```python
from build123d import *

# Parameters (mm, degrees)
F0_R      = 15.5
F1_DEPTH  = 57.2
F3_DEPTH  = 58.1
F4_R      = 9.45
F5_DEPTH  = 3.5
F5_FACE_R = 9.45
F6_DEPTH  = 34
F7_R      = 4
F8_DEPTH  = 16
F9_R      = 4
F9_R_2    = 2
F10_DEPTH = 2
F11_DEPTH = 29
F12_R     = 6
F13_DEPTH = 2


with BuildPart() as f1:
    # F0 (on Top) → F1 (new body)
    with BuildSketch(Plane.XY):
        Circle(F0_R)
    extrude(amount=F1_DEPTH)

    # F2 (on face) → F3 (join)
    with BuildSketch(Plane.XY.offset(57.2)):
        with BuildLine():
            Line((-12.208501, 9.55), (-20.06, 9.55))
            Line((-20.06, 9.55), (-20.06, -17.45))
            Line((-20.06, -17.45), (20.06, -17.45))
            Line((20.06, -17.45), (20.06, 9.55))
            Line((20.06, 9.55), (12.208501, 9.55))
            ThreePointArc((12.208501, 9.55), (14.65404, 5.050655), (15.5, 0))
            ThreePointArc((15.5, 0), (-5.050655, -14.65404), (-12.208501, 9.55))
        make_face()
        with BuildLine():
            Line((12.208501, 9.55), (-12.208501, 9.55))
            ThreePointArc((-12.208501, 9.55), (-5.050655, -14.65404), (15.5, 0))
            ThreePointArc((15.5, 0), (14.65404, 5.050655), (12.208501, 9.55))
        make_face()
    extrude(amount=F3_DEPTH)

    # F4 (on face) → F5 (join)
    with BuildSketch(Plane.XZ.offset(17.45)):
        with Locations((0, 95.1)):
            Circle(F4_R)
    extrude(amount=F5_DEPTH)

    # F5_face (on face) → F6 (join)
    with BuildSketch(Plane(origin=(0, -20.95, 95.1), x_dir=(1, 0, 0), z_dir=(0, -1, 0))):
        Circle(F5_FACE_R)
    extrude(amount=-F6_DEPTH)

    # F7 (on face) → F8 (join)
    with BuildSketch(Plane.XZ.offset(20.95)):
        with Locations((0, 95.1)):
            Circle(F7_R)
    extrude(amount=F8_DEPTH)

    # F9 (on face) → F10 (join)
    with BuildSketch(Plane.XZ.offset(17.45)):
        with Locations((14, 106.25)):
            Circle(F9_R)
        with Locations((14, 106.25)):
            Circle(F9_R_2, mode=Mode.SUBTRACT)
        with Locations((-14, 106.25)):
            Circle(F9_R)
        with Locations((-14, 106.25)):
            Circle(F9_R_2, mode=Mode.SUBTRACT)
        with Locations((14, 66.25)):
            Circle(F9_R)
        with Locations((14, 66.25)):
            Circle(F9_R_2, mode=Mode.SUBTRACT)
        with Locations((-14, 66.25)):
            Circle(F9_R)
        with Locations((-14, 66.25)):
            Circle(F9_R_2, mode=Mode.SUBTRACT)
    extrude(amount=F10_DEPTH)

    # F9 (on face) → F11 (join)
    with BuildSketch(Plane.XZ.offset(17.45)):
        with Locations((14, 106.25)):
            Circle(F9_R)
        with Locations((14, 106.25)):
            Circle(F9_R_2, mode=Mode.SUBTRACT)
        with Locations((-14, 106.25)):
            Circle(F9_R)
        with Locations((-14, 106.25)):
            Circle(F9_R_2, mode=Mode.SUBTRACT)
        with Locations((14, 66.25)):
            Circle(F9_R)
        with Locations((14, 66.25)):
            Circle(F9_R_2, mode=Mode.SUBTRACT)
        with Locations((-14, 66.25)):
            Circle(F9_R)
        with Locations((-14, 66.25)):
            Circle(F9_R_2, mode=Mode.SUBTRACT)
    extrude(amount=-F11_DEPTH)

    # F12 (on face) → F13 (join)
    with BuildSketch(Plane(origin=(0, 0, 0), x_dir=(1, 0, 0), z_dir=(0, 0, -1))):
        Circle(F12_R)
    extrude(amount=F13_DEPTH)


solid = f1.part
```
Geometry: final body of the model. Coordinates: model frame, mm. A direction names the side the tool comes from. Coordinates: 2 decimals unless noted, no trailing zeros. Order: outer loops, then holes, each group sorted by start corner. A loop starts at its lowest first (then second) coordinate and runs counter-clockwise, first axis right, second up. Notation, with made-up numbers: M -22.75,56 L 16.25,56 A16 ccw 16.25,68 Z; hole C 45,5 d9. An arc over 180 degrees is marked long. Answer in a Markdown table with one row per item. Add a question column.
Q1. Mould query, pull axis Z, two halves, no side actions, for faces 6 (the flat face through (0, 13.05, 95)), 7 (the cylindrical face through (-17.996, 10.536, 106.426)), 8 (the flat face through (0, -7, 0)). Classes: released by +Z, released by -Z, zero draft, split by the parting line, or undercut.
Q2. Line query: L1, parallel to Z at x = -14, y = -18.05; L2, parallel to X at y = -18, z = 66; L3, parallel to Y at x = -13, z = 61. Output: solid intervals per line, ascending.
Q3. Section query A-A on x = 0. Return the cut outline in (y, z), and give its area (3 significant figures).
Q4. Reachability of faces 1 (the cylindrical face through (-6, 0, -1)), 2 (the cylindrical face through (-14.867, -18.436, 62.345)), 3 (the flat face through (0, -36.95, 95)), 4 (the cylindrical face through (13.74, 10.536, 68.233)), 5 (the flat face through (20.06, -4, 86)) from +Z, -Z, +X, -X, +Y, -Y: full face, straight path, thin tool, end or side. Return the list, or none.
Q5. Section query B-B on y = -9.5. Return the cut outline in (x, z), and give its area (3 significant figures).
Q6. Section query C-C on z = 81. Return the cut outline in (x, y), and give its area (3 significant figures).
Q7. Section query D-D on y = 0. Return the cut outline in (x, z), and give its area (3 significant figures).
Q8. Contact query for flat-ended pins moving along their axis: P1, Ø5, axis at x = 10, z = 99.5, coming from the +Y side; P2, Ø3, axis at x = 14, z = 66.25, coming from the +Y side; P3, Ø9, axis at x = -14, z = 106, coming from the +Y side; P4, Ø10, axis at x = -11, y = -29, coming from the -Z side. Output: stop coordinate, or through.
Completed:
| question | item | result |
|---|---|---|
| 1 | face 6 | zero draft |
| 1 | face 7 | undercut |
| 1 | face 8 | released by -Z |
| 2 | L1 | z = 62.25 to 64.25, 68.25 to 70.25, 102.25 to 104.25, 108.25 to 110.25 |
| 2 | L2 | x = -17.99 to -15.98, -12.02 to -10.01, 10.01 to 12.02, 15.98 to 17.99 |
| 2 | L3 | y = -17.45 to 9.55 |
| 3 | outline | M -36.95,91.1 L -20.95,91.1 L -20.95,85.65 L -17.45,85.65 L -17.45,57.2 L -15.5,57.2 L -15.5,0 L -6,0 L -6,-2 L 6,-2 L 6,0 L 15.5,0 L 15.5,57.2 L 9.55,57.2 L 9.55,85.65 L 13.05,85.65 L 13.05,104.55 L 9.55,104.55 L 9.55,115.3 L -17.45,115.3 L -17.45,104.55 L -20.95,104.55 L -20.95,99.1 L -36.95,99.1 Z |
| 3 | area | 3,630 mm2 |
| 4 | face 1 | -Z |
| 4 | face 2 | -Y |
| 4 | face 3 | +Z, -Z, +X, -X, -Y |
| 4 | face 4 | +Y |
| 4 | face 5 | +Z, -Z, +X, +Y, -Y |
| 5 | outline | M -20.06,57.2 L -12.25,57.2 L -12.25,0 L 12.25,0 L 12.25,57.2 L 20.06,57.2 L 20.06,115.3 L -20.06,115.3 Z |
| 5 | area | 3,730 mm2 |
| 6 | outline | M -20.06,-17.45 L 20.06,-17.45 L 20.06,9.55 L -20.06,9.55 Z |
| 6 | area | 1,080 mm2 |
| 7 | outline | M -20.06,57.2 L -15.5,57.2 L -15.5,0 L -6,0 L -6,-2 L 6,-2 L 6,0 L 15.5,0 L 15.5,57.2 L 20.06,57.2 L 20.06,115.3 L -20.06,115.3 Z |
| 7 | area | 4,130 mm2 |
| 8 | P1 | stops at y = 13.05 |
| 8 | P2 | stops at y = 9.55 |
| 8 | P3 | stops at y = 11.55 |
| 8 | P4 | passes through |
